Read the model definition and answer for the solid it produces. Units are mm, in the model's axes. A direction names the side the tool comes from. Round coordinates to 2 decimals unless told otherwise and drop trailing zeros. Order: outer loops, then holes, each group sorted by start corner. A loop starts at its lowest first (then second) coordinate and runs counter-clockwise, first axis right, second up. Notation, with made-up numbers: M 62,82.5 L 96,82.5 A26 ccw 96,112.5 Z; hole C -30,38.25 d4. An arc over 180 degrees is marked long. Answer as CSV lines item,"result".
Solid Edge part; units mm, degrees
sketch "Sketch1" plane through (0, 0, 0) normal (0, 0, 1) x (1, 0, 0)
  line L0 (-2.3094, 4) -> (2.3094, 4)
  line L1 (2.3094, 4) -> (4.6188, 0)
  line L2 (4.6188, 0) -> (2.3094, -4)
  line L3 (2.3094, -4) -> (-2.3094, -4)
  line L4 (-2.3094, -4) -> (-4.6188, 0)
  line L5 (-4.6188, 0) -> (-2.3094, 4)
extrude "Protrusion1" add sketch "Sketch1" along normal blind 0.5
sketch "Sketch2" plane through (0, 0, 0.5) normal (0, 0, 1) x (1, 0, 0)
  circle A0 centre (0, 0) radius 3.5
extrude "Ausprägung_2" add sketch "Sketch2" along normal blind 5.5
hole "Bohrung_1" at (0, 0, 6) direction (0, 0, -1) diameter 4 depth 4
chamfer "Fase_1" distance 0.5 angle 45 1 edges at (0, 2, 6)
Item 1: A cutting plane is placed at B-B, the plane z = 1.65. Determine the outline of the cut face in (x, y), and give its area (3 significant figures).
Ans:
outline,"C 0,0 d7"
area,"38.5 mm2"
Item 2: Flat-ended cylindrical pins translate along their axes: pin 1 (1.2 mm diameter, centred on x = -1, y = -0.5, fed in from +Z); pin 2 (3 mm diameter, centred on y = 0, z = 5, fed in from +X); pin 3 (1 mm diameter, centred on x = 3, z = 2, fed in from -Y). Find the tip coordinate at first contact, or state that the pin passes through.
Ans:
pin 1,"z = 2"
pin 2,"x = 3.5"
pin 3,"y = -2.45"
Item 3: A cutting plane is placed at C-C, the plane x = 3.25. Determine the outline of the cut face in (y, z).
Ans:
outline,"M -2.37,0 L 2.37,0 L 2.37,0.5 L 1.3,0.5 L 1.3,6 L -1.3,6 L -1.3,0.5 L -2.37,0.5 Z"
Item 4: A cutting plane is placed at A-A, the plane x = 0. Determine the outline of the cut face in (y, z), and give its area (4 significant figures).
Ans:
outline,"M -4,0 L 4,0 L 4,0.5 L 3.5,0.5 L 3.5,6 L 2.5,6 L 2,5.5 L 2,2 L -2,2 L -2,5.5 L -2.5,6 L -3.5,6 L -3.5,0.5 L -4,0.5 Z"
area,"26.25 mm2"
Item 5: A tool of negligible diameter and unlimited length cuts with its end or side. For faces 1 (the face through (-3.48, 1.97, 0.25)), 2 (the face through (2, 0, 4)), from which of +Z, -Z, +X, -X, +Y, -Y can it reach the whole face along a straight path? Write none if from no direction.
Ans:
face 1,"+Z, -Z, -X, +Y"
face 2,"+Z"
Item 6: Find the intervals of material crossed by probe 1 along Y at (x, z) = (0, 3.45); probe 2 along Z at (x, y) = (-2, -3.25); probe 3 along Y at (x, z) = (-1.5, 2.45), in increasing order. Write a range as [from, to].
Ans:
probe 1,"[-3.5, -2], [2, 3.5]"
probe 2,"[0, 0.5]"
probe 3,"[-3.16, -1.32], [1.32, 3.16]"
Item 7: Determine the mould class of faces 3 (the face through (3.448, 2.028, 0.246)), 4 (the face through (0, 0, 2)), 5 (the face through (0, 0, 0)) for opening direction X: +X half, -X half, draft (parallel to the pull), parting line (faces both ways), or undercut.
Ans:
face 3,"+X half"
face 4,"undercut"
face 5,"draft"
